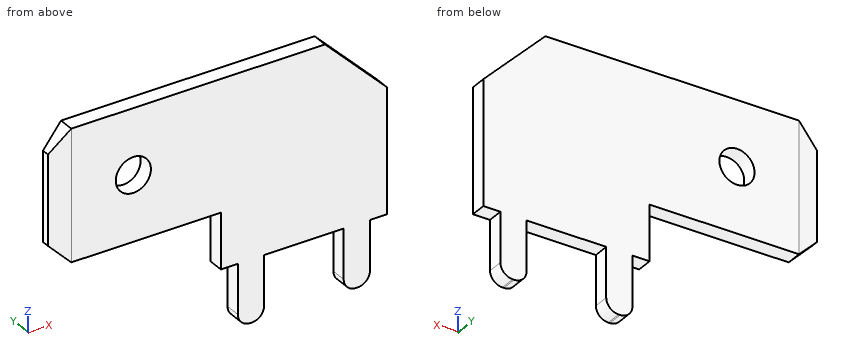
```python
from build123d import *

# Parameters (mm, degrees)
F1_DEPTH = 0.385
F2_SIZE  = 1
F3_R     = 0.85
F4_DEPTH = 0.771
F6_DEPTH = 12.001


with BuildPart() as f1:
    # F0 (on Front) → F1 (new body, symmetric)
    with BuildSketch(Plane.XZ):
        with BuildLine():
            Line((-4.02, 2.68), (-4.02, 0))
            Line((-4.02, 0), (-3.195, 0))
            Line((-3.195, 0), (-3.195, -2.4))
            ThreePointArc((-3.195, -2.4), (-3.019264, -2.824264), (-2.595, -3))
            Line((-2.595, -3), (-2.525, -3))
            ThreePointArc((-2.525, -3), (-2.100736, -2.824264), (-1.925, -2.4))
            Line((-1.925, -2.4), (-1.925, 0))
            Line((-1.925, 0), (1.925, 0))
            Line((1.925, 0), (1.925, -2.4))
            ThreePointArc((1.925, -2.4), (2.100736, -2.824264), (2.525, -3))
            Line((2.525, -3), (2.595, -3))
            ThreePointArc((2.595, -3), (3.019264, -2.824264), (3.195, -2.4))
            Line((3.195, -2.4), (3.195, 0))
            Line((3.195, 0), (4.02, 0))
            Line((4.02, 0), (4.02, 6))
            Line((4.02, 6), (1.02, 9))
            Line((1.02, 9), (-11.25, 9))
            Line((-11.25, 9), (-12.25, 9))
            Line((-12.25, 9), (-12.25, 2.68))
            Line((-12.25, 2.68), (-11.25, 2.68))
            Line((-11.25, 2.68), (-4.02, 2.68))
        make_face()
    extrude(amount=F1_DEPTH, both=True)

    # F2
    f2_edges = [f1.edges().sort_by_distance(p)[0] for p in [
        (-12.25, 0, 9),
        (-12.25, 0, 2.68),
    ]]
    chamfer(f2_edges, length=F2_SIZE)

    # F3 (on face) → F4 (cut, through all)
    with BuildSketch(Plane.XZ.offset(0.385)):
        with Locations((-8.25, 5.84)):
            Circle(F3_R)
    extrude(amount=-F4_DEPTH, mode=Mode.SUBTRACT)

    # F5 (on face) → F6 (cut, through all)
    with BuildSketch(Plane.XY.offset(9)):
        Polygon((-12.25, 0.185), (-11.25, 0.385), (-12.25, 0.385), align=None)
        Polygon((-12.25, -0.385), (-11.25, -0.385), (-12.25, -0.185), align=None)
    extrude(amount=-F6_DEPTH, mode=Mode.SUBTRACT)


solid = f1.part
```
Source: CAD feature listing. Evaluate the final solid. Frame: model axes, mm. Round coordinates to 2 decimals unless told otherwise and drop trailing zeros. Order: outer loops, then holes, each group sorted by start corner. A loop starts at its lowest first (then second) coordinate and runs counter-clockwise, first axis right, second up. Notation, with made-up numbers: (61, -22.75) -> (68, -22.75) arc R16 ccw to (68, -4.75) -> close; hole circle Ø2 at (57.5, -21). An arc over 180 degrees is marked (long way). Use CSV: the item, a comma, the result in double quotes.
(1) Section A-A on x = -8.25. Return the cut outline in (y, z) (3 decimals).
Report:
outline,"(-0.385, 2.68) -> (0.385, 2.68) -> (0.385, 4.99) -> (-0.385, 4.99) -> close; (-0.385, 6.69) -> (0.385, 6.69) -> (0.385, 9) -> (-0.385, 9) -> close"
(2) Ray query, L1, parallel to Z at x = -8.25, y = 0.1; L2, parallel to X at y = -0.15, z = -1.5 (3 decimals); L3, parallel to X at y = -0.2, z = 1. Return the intervals inside material, ascending.
Report:
L1,"2.68 to 4.99, 6.69 to 9"
L2,"-3.195 to -1.925, 1.925 to 3.195"
L3,"-4.02 to 4.02"
(3) Section B-B on z = -1. Return the cut outline in (x, y) (3 decimals), and give its area (3 significant figures).
Report:
outline,"(-3.195, -0.385) -> (-1.925, -0.385) -> (-1.925, 0.385) -> (-3.195, 0.385) -> close; (1.925, -0.385) -> (3.195, -0.385) -> (3.195, 0.385) -> (1.925, 0.385) -> close"
area,"1.96 mm^2"
(4) Section C-C on z = 3.25. Return the cut outline in (x, y) (3 decimals).
Report:
outline,"(-11.82, -0.271) -> (-11.25, -0.385) -> (4.02, -0.385) -> (4.02, 0.385) -> (-11.25, 0.385) -> (-11.82, 0.271) -> close"
(5) Section D-D on x = -11. Return the cut outline in (y, z) (3 decimals), and give its area (3 significant figures).
Report:
outline,"(-0.385, 2.68) -> (0.385, 2.68) -> (0.385, 9) -> (-0.385, 9) -> close"
area,"4.87 mm^2"
